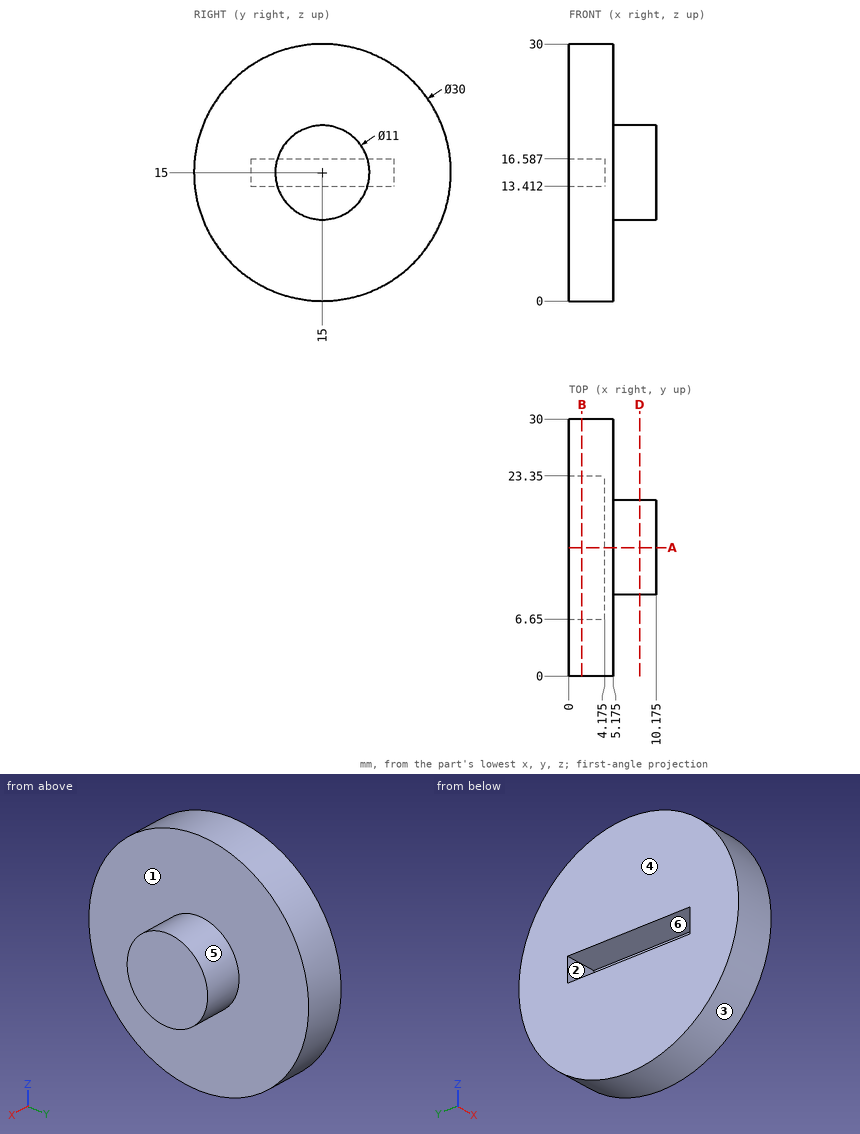
Job drawing, mm, ordinate dimensions from the low corner. One solid piece. A direction names the side the tool comes from. Round coordinates to 2 decimals unless told otherwise and drop trailing zeros. Order: outer loops, then holes, each group sorted by start corner. A loop starts at its lowest first (then second) coordinate and runs counter-clockwise, first axis right, second up. Notation, with made-up numbers: M 61,61 L 70,61 A7 ccw 70,74 Z; hole C 71,74.5 d9. An arc over 180 degrees is marked long. Write each question's results on one line, items separated by ' | '. Start each with the question number.
(1) Saw through at A-A, the plane y = 15. Give the cut face in (x, z) (1 decimal), then the cut area to 3 significant figures.
(2) Two-plate mould, pull along Z, no slides. Class the marked faces 4, 5 and 6: pulls with the +Z half, pulls with the -Z half, needs draft (parallel to the pull), parting line crosses it, or undercut.
(3) Drop flat-ended pins along their axis: pin 1 (5 mm diameter, centred on x = 6, y = 23.5, fed in from +Z) (1 decimal); pin 2 (4.5 mm diameter, centred on x = 1, y = 18, fed in from +Z); pin 3 (3 mm diameter, centred on x = 6, z = 22, fed in from +Y) (1 decimal). Give the stop position or say it passes through.
(4) Which spindle directions (+Z, -Z, +X, -X, +Y, -Y) get a long thin tool onto all of the face, cutting with end or side? Do the marked faces 1, 2 and 3. Say none if no direction does.
(5) Saw through at B-B, the plane x = 1.5. Give the cut face in (y, z).
(6) Probe probe 1 along Z at (x, y) = (7.25, 15.25) (1 decimal); probe 2 along X at (y, z) = (26.5, 14) (1 decimal); probe 3 along Z at (x, y) = (0.5, 23). List the from-to ranges inside material, lowest first. Write a range as from..to.
(7) Saw through at D-D, the plane x = 8.25. Give the cut face in (y, z).
Established:
1) outline: M 0,0 L 5.2,0 L 5.2,9.5 L 10.2,9.5 L 10.2,20.5 L 5.2,20.5 L 5.2,30 L 0,30 L 0,16.6 L 4.2,16.6 L 4.2,13.4 L 0,13.4 Z | area: 197 mm^2
2) face 4: needs draft | face 5: parting line crosses it | face 6: undercut
3) pin 1: stops at z = 28.7 | pin 2: stops at z = 29.98 | pin 3: stops at y = 28.9
4) face 1: +X | face 2: -X | face 3: +X, -X
5) outline: C 15,15 d30; hole M 6.65,13.41 L 23.35,13.41 L 23.35,16.59 L 6.65,16.59 Z
6) probe 1: z = 9.5..20.5 | probe 2: x = 0..5.2 | probe 3: z = 2.31..13.41, 16.59..27.69
7) outline: C 15,15 d11
